from build123d import *

# Parameters (mm, degrees)
CROQUIS1_W                                   = 70
CROQUIS1_H                                   = 30
SALIENTE_EXTRUIR1_DEPTH                      = 3
SALIENTE_EXTRUIR2_DEPTH                      = 24
CORTAR_EXTRUIR1_DEPTH                        = 70.000004
CROQUIS5_R                                   = 1.5
CORTAR_EXTRUIR2_DEPTH                        = 3
REFRENTADO_PARA_TORNILLO_TAP_N_CON_C_2_COUNT = 2
REFRENTADO_PARA_TORNILLO_TAP_N_CON_C_2_PITCH = 30
REDONDEO1_R                                  = 5


with BuildPart() as part:
    # Croquis1 → Saliente-Extruir1 (new body)
    with BuildSketch(Plane.XY):
        with Locations((5.076335878, 0.496183206)):
            Rectangle(CROQUIS1_W, CROQUIS1_H)
    extrude(amount=SALIENTE_EXTRUIR1_DEPTH)

    # Croquis3 → Saliente-Extruir2 (add)
    with BuildSketch(Plane.XY.offset(3)):
        Polygon((-29.923664122, 0.496183206), (40.076335878, 0.496183206), (40.076335878, -4.503816794), (40.076335878, -14.503816794), (36.076335878, -14.503816794), (36.076335878, -4.503816794), (18.076335878, -4.503816794), (18.076335878, -14.503816794), (14.076335878, -14.503816794), (14.076335878, -4.503816794), (-3.923664122, -4.503816794), (-3.923664122, -14.503816794), (-7.923664122, -14.503816794), (-7.923664122, -4.503816794), (-25.923664122, -4.503816794), (-25.923664122, -14.503816794), (-29.923664122, -14.503816794), (-29.923664122, -4.503816794), align=None)
    extrude(amount=SALIENTE_EXTRUIR2_DEPTH)

    # Croquis4 → Cortar-Extruir1 (cut)
    with BuildSketch(Plane.ZY.offset(29.923664122)):
        with BuildLine():
            Line((27, -14.503816794), (27, -4.503816794))
            ThreePointArc((27, -4.503816794), (14.366976751, -7.984560996), (3, -14.503816794))
            Line((3, -14.503816794), (27, -14.503816794))
        make_face()
    extrude(amount=-CORTAR_EXTRUIR1_DEPTH, mode=Mode.SUBTRACT)

    # Croquis5 → Cortar-Extruir2 (cut)
    with BuildSketch(Plane.XY.offset(3)):
        with Locations((-9.923664122, 7.996183206)):
            Circle(CROQUIS5_R)
        with Locations(Location((20.076335878, 7.996183206, 0), (0, 0, 180))):
            Circle(CROQUIS5_R)
    extrude(amount=-CORTAR_EXTRUIR2_DEPTH, mode=Mode.SUBTRACT)

    # Croquis7 → Refrentado para tornillo tapón con cabeza plana de clavija de M31 (revolve, cut)
    with BuildSketch(Plane(origin=(-9.923664122, 7.996183206, 3), x_dir=(0, -1, 0), z_dir=(1, 0, 0))):
        Polygon((0, 0), (0, 3), (1.7, 3), (1.7, 1.66), (3.36, 0), align=None)
    refrentado_para_tornillo_tap_n_con_cabez = revolve(axis=Axis((-9.923664122, 7.996183206, 9.35), (0, 0, -1)), mode=Mode.SUBTRACT)

    # Refrentado para tornillo tap_n con c 2: Refrentado para tornillo tapón con cabeza plana de clavija de M31 ×2
    with Locations(*[(i * REFRENTADO_PARA_TORNILLO_TAP_N_CON_C_2_PITCH, 0, 0) for i in range(1, REFRENTADO_PARA_TORNILLO_TAP_N_CON_C_2_COUNT)]):
        add(refrentado_para_tornillo_tap_n_con_cabez, mode=Mode.SUBTRACT)

    # Redondeo1
    # the kernel refuses this fillet: 5 mm, written as the material it takes off along each edge
    with BuildSketch(Plane(origin=(40.076335878, -14.503816794, 15.5), x_dir=(0, 1, 0), z_dir=(0, 0, -1)), Plane(origin=(-29.923664122, -14.503816794, -12.5), x_dir=(0, 1, 0), z_dir=(0, 0, 1)), Plane(origin=(-29.923664122, 15.496183206, -12.5), x_dir=(1, 0, 0), z_dir=(0, 0, 1))) as redondeo1_piece_1:
        with BuildLine():
            CenterArc((REDONDEO1_R, -REDONDEO1_R), REDONDEO1_R, 90, 90)
            Line((0, -REDONDEO1_R), (0, 0))
            Line((0, 0), (REDONDEO1_R, 0))
        make_face()
    extrude(amount=28, mode=Mode.SUBTRACT)
    with BuildSketch(Plane(origin=(40.076335878, 15.496183206, -12.5), x_dir=(-1, 0, 0), z_dir=(0, 0, 1))) as redondeo1_piece_2:
        with BuildLine():
            CenterArc((REDONDEO1_R, REDONDEO1_R), REDONDEO1_R, 180, 90)
            Line((0, REDONDEO1_R), (0, 0))
            Line((0, 0), (REDONDEO1_R, 0))
        make_face()
    extrude(amount=28, mode=Mode.SUBTRACT)


solid = part.part
Work out the finished part from the listing and answer in its coordinate system (mm). A direction names the side the tool comes from. Coordinates: 2 decimals unless noted, no trailing zeros. Loops run counter-clockwise (first coordinate to the right, second up) from the corner with the lowest first, then second, coordinate; pieces in that order, holes last. Notation, with made-up numbers: (18, 61) -> (28, 61) arc R26 cw to (28, 76) -> close; hole circle Ø3 at (-36.75, 24). An arc over 180 degrees is marked (long way). Write each question's results on one line, items separated by ' | '. Start each with the question number.
1) Find section B-B on y = -8. Determine the outline of the cut face in (x, z), then the cut area to 3 significant figures.
2) Find section D-D on y = 8. Count the separate pieces of the cut face and the enclosed holes in it, then the cut area to 3 significant figures.
3) Consider line 1 along X through (y, z) = (-8.5, 6); line 2 along Z through (x, y) = (35, 1.5); line 3 along Y through (x, z) = (-13.5, 13). Determine where each line is inside the solid, lowest interval first.
4) Find section A-A on x = 0. Determine the outline of the cut face in (y, z).
5) Flat-ended cylindrical pins translate along their axes: P1, Ø1, axis at y = -11.5, z = 4.5, coming from the +X side; P2, Ø2, axis at x = -9.92, y = 8, coming from the +Z side; P3, Ø3, axis at x = 31, y = -10.5, coming from the +Z side; P4, Ø4, axis at x = -21.5, z = 8, coming from the -Y side. Find the tip coordinate at first contact, or state that the pin passes through.
6) The mould has two halves that part along X. Classify faces 1 (the flat face through (-7.924, -7, 9)), 2 (the cylindrical face through (-29.05, -12.33, 2.99)), 3 (the cylindrical face through (-5.952, -7.914, 14.537)), 4 (the flat face through (40.076, -2, 10)): pulls with the +X half, pulls with the -X half, needs draft (parallel to the pull), parting line crosses it, or undercut.
7) For faces 5 (the flat face through (5, 0.496, 15)), 6 (the flat face through (14.076, -7, 9)), 7 (the flat face through (5, 1, 0)), determine the directions among +Z, -Z, +X, -X, +Y, -Y from which every point of the face is accessible in a straight line to the end or side of a thin tool.
8) Find section C-C on z = 11.75. Determine the outline of the cut face in (x, y).
Response values:
1) outline: (-29.92, 0) -> (40.08, 0) -> (40.08, 14.33) -> (36.08, 14.33) -> (36.08, 3) -> (18.08, 3) -> (18.08, 14.33) -> (14.08, 14.33) -> (14.08, 3) -> (-3.92, 3) -> (-3.92, 14.33) -> (-7.92, 14.33) -> (-7.92, 3) -> (-25.92, 3) -> (-25.92, 14.33) -> (-29.92, 14.33) -> close | area: 391 mm^2
2) separate pieces: 3 | enclosed holes: 0 | area: 184 mm^2
3) line 1: x = -29.92 to -25.92, -7.92 to -3.92, 14.08 to 18.08, 36.08 to 40.08 | line 2: z = 0 to 3 | line 3: y = -4.5 to 0.5
4) outline: (-14.5, 0) -> (15.5, 0) -> (15.5, 3) -> (0.5, 3) -> (0.5, 27) -> (-4.5, 27) -> (-4.5, 3) -> (-14.5, 3) -> close
5) P1: stops at x = 39.85 | P2: passes through | P3: stops at z = 3 | P4: stops at y = -4.5
6) face 1: undercut | face 2: pulls with the -X half | face 3: needs draft | face 4: pulls with the +X half
7) face 5: +Z, +X, -X, +Y | face 6: +Z, -Y | face 7: -Z, +X, -X, +Y, -Y
8) outline: (-29.92, -9.16) -> (-25.92, -9.16) -> (-25.92, -4.5) -> (-7.92, -4.5) -> (-7.92, -9.16) -> (-3.92, -9.16) -> (-3.92, -4.5) -> (14.08, -4.5) -> (14.08, -9.16) -> (18.08, -9.16) -> (18.08, -4.5) -> (36.08, -4.5) -> (36.08, -9.16) -> (40.08, -9.16) -> (40.08, 0.5) -> (-29.92, 0.5) -> close
